Drawing for the job (mm, zero at the part's lowest x, y, z). A direction names the side the tool comes from. Round coordinates to 2 decimals unless told otherwise and drop trailing zeros. Write each loop counter-clockwise with the first axis right and the second up, starting at its lowest first coordinate (ties: lowest second). Pieces come first, ordered by that corner, then holes. Notation, with made-up numbers: M -12,65.25 L 24,65.25 A18 ccw 24,92.25 Z; hole C -32,56.5 d4. An arc over 180 degrees is marked long. Use a Markdown table: item, result.
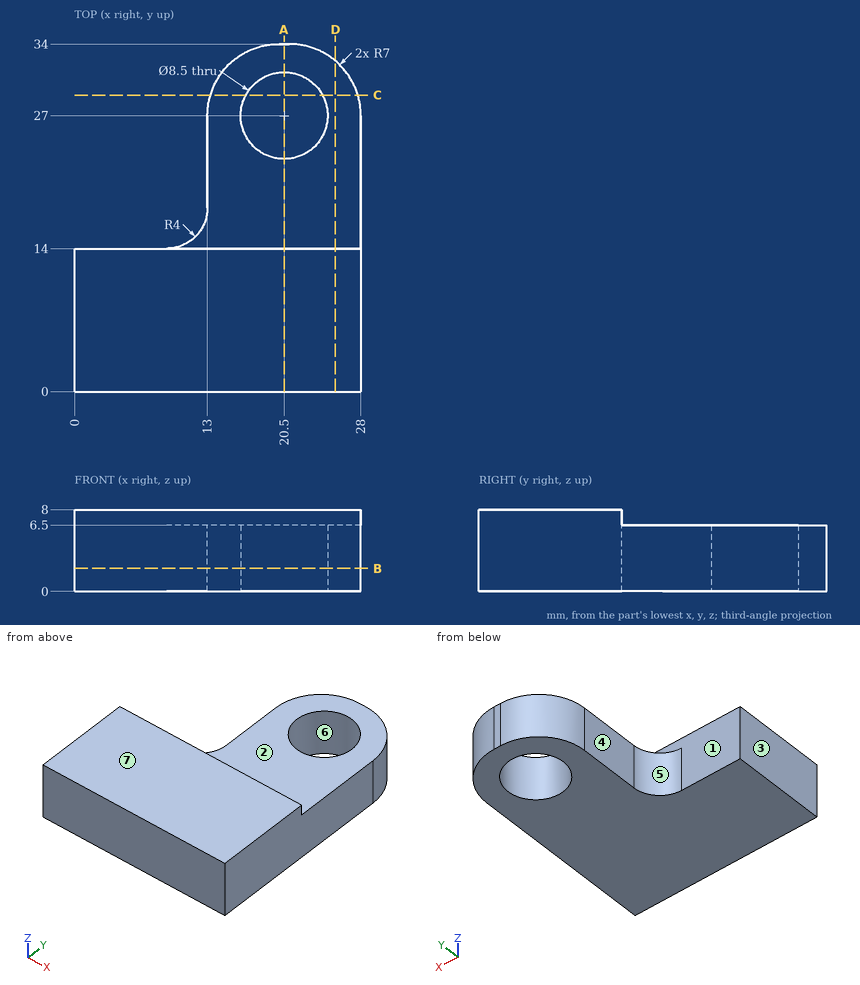
Q1. Cut at C-C on y = 29. Give the cut face in (x, z).
Response values:
| item | result |
|---|---|
| outline | M 13.29,0 L 16.75,0 L 16.75,6.5 L 13.29,6.5 Z; M 24.25,0 L 27.71,0 L 27.71,6.5 L 24.25,6.5 Z |
Q2. Two-plate mould, pull along Y, no slides. Class the marked faces 5, 6 and 7: +Y half, -Y half, draft (parallel to the pull), parting line (faces both ways), or undercut.
Response values:
| item | result |
|---|---|
| face 5 | +Y half |
| face 6 | undercut |
| face 7 | draft |
Q3. Drop flat-ended pins along their axis: P1, Ø3, axis at y = 20.5, z = 3.5, coming from the -X side; P2, Ø4, axis at x = 16.5, z = 3.5, coming from the +Y side. Give the stop position or say it passes through.
Response values:
| item | result |
|---|---|
| P1 | stops at x = 13 |
| P2 | stops at y = 33.84 |
Q4. Cut at A-A on x = 20.5. Give the cut face in (y, z), and give its area (3 significant figures).
Response values:
| item | result |
|---|---|
| outline | M 0,0 L 22.75,0 L 22.75,6.5 L 14,6.5 L 14,8 L 0,8 Z; M 31.25,0 L 34,0 L 34,6.5 L 31.25,6.5 Z |
| area | 187 mm2 |
Q5. Cut at B-B on z = 2.25. Give the cut face in (x, y), and give its area (3 significant figures).
Response values:
| item | result |
|---|---|
| outline | M 0,0 L 28,0 L 28,27 A7 ccw 21,34 L 20,34 A7 ccw 13,27 L 13,18 A4 cw 9,14 L 0,14 Z; hole C 20.5,27 d8.5 |
| area | 618 mm2 |
Q6. Which spindle directions (+Z, -Z, +X, -X, +Y, -Y) get a long thin tool onto all of the face, cutting with end or side? Do the marked faces 1, 2, 3 and 4. Say none if no direction does.
Response values:
| item | result |
|---|---|
| face 1 | +Z, -X, +Y |
| face 2 | +Z, +X, -X, +Y |
| face 3 | +Z, -Z, -X, +Y, -Y |
| face 4 | +Z, -Z, -X, +Y |
Q7. Cut at D-D on x = 25.5. Give the cut face in (y, z), and give its area (3 significant figures).
Response values:
| item | result |
|---|---|
| outline | M 0,0 L 32.36,0 L 32.36,6.5 L 14,6.5 L 14,8 L 0,8 Z |
| area | 231 mm2 |
Q8. Drill centre lines: L1, parallel to X at y = 27, z = 4.25; L2, parallel to Y at x = 20.5, z = 1.75; L3, parallel to Y at x = 24, z = 1. Where is each one in solid material? Low to high.
Response values:
| item | result |
|---|---|
| L1 | x = 13 to 16.25, 24.75 to 28 |
| L2 | y = 0 to 22.75, 31.25 to 34 |
| L3 | y = 0 to 24.59, 29.41 to 33.32 |
